from build123d import *

# Parameters (mm, degrees)
F0_W           = 80
F0_H           = 80
F1_DEPTH       = 7
F3_D           = 7.5
F4_R           = 6
F5_SIZE        = 25
F6_SIZE        = 20
F8_D           = 5.5
F8_CBORE_D     = 10
F8_CBORE_DEPTH = 3
F9_R           = 10
F10_D          = 5.5


with BuildPart() as f1:
    # F0 (on Top) → F1 (new body)
    with BuildSketch(Plane.XY):
        Rectangle(F0_W, F0_H)
    extrude(amount=F1_DEPTH)

    # F3 (through all)
    with Locations(Plane.XY.offset(7)):
        with Locations((0, -30)):
            Hole(F3_D / 2)

    # F4
    f4_edges = [f1.edges().sort_by_distance(p)[0] for p in [
        (-40, 40, 3.5),
        (40, 40, 3.5),
    ]]
    fillet(f4_edges, radius=F4_R)

    # F5
    f5_edges = [f1.edges().sort_by_distance(p)[0] for p in [
        (-40, -40, 3.5),
        (40, -40, 3.5),
    ]]
    chamfer(f5_edges, length=F5_SIZE)

    # F6
    f6_edges = [f1.edges().sort_by_distance(p)[0] for p in [
        (40, -15, 3.5),
        (-40, -15, 3.5),
    ]]
    chamfer(f6_edges, length=F6_SIZE)

    # F8 (through all)
    with Locations(Plane.XY.offset(7)):
        with Locations((-20, 20), (0, 20), (20, 20), (20, 0), (0, 0), (-20, 0)):
            CounterBoreHole(F8_D / 2, F8_CBORE_D / 2, F8_CBORE_DEPTH)

    # F9
    f9_edges = [f1.edges().sort_by_distance(p)[0] for p in [
        (40, 5, 3.5),
        (25.857864, -29.142136, 3.5),
        (15, -40, 3.5),
        (-15, -40, 3.5),
        (-40, 5, 3.5),
        (-25.857864, -29.142136, 3.5),
    ]]
    fillet(f9_edges, radius=F9_R)

    # F10 (through all)
    with Locations(Plane.XY.offset(7)):
        with Locations((-30, 30), (30, 30)):
            Hole(F10_D / 2)


solid = f1.part
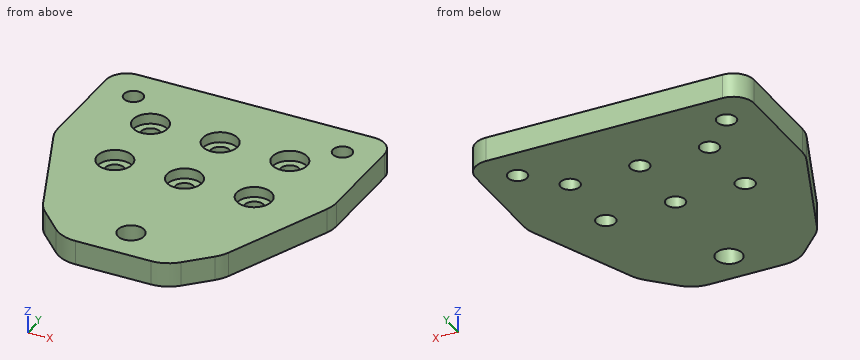
Geometry: final body of the model. Coordinates: model frame, mm. Give positions to 0.01 mm unless a question says otherwise; leave off trailing zeros. Order: outer loops, then holes, each group sorted by start corner. A loop starts at its lowest first (then second) coordinate and runs counter-clockwise, first axis right, second up. Notation, with made-up numbers: (17, 81.5) -> (56, 81.5) arc R23 ccw to (56, 113.5) -> close; hole circle Ø9 at (-34, 18.25). An arc over 180 degrees is marked (long way). Answer as a JSON object with one key per item and string values.
Q1. Section B-B (z = 1.75). State how many separate pieces and enclosed holes the cut face has, plus the area to 3 significant figures.
Entries:
{"separate pieces": "1", "enclosed holes": "9", "area": "5,240 mm^2"}
Q2. Section D-D (x = 0). Output: boundary loops of the cut face in (y, z), plus the area to 4 significant figures.
Entries:
{"outline": "(-40, 0) -> (-33.75, 0) -> (-33.75, 7) -> (-40, 7) -> close; (-26.25, 0) -> (-2.75, 0) -> (-2.75, 4) -> (-5, 4) -> (-5, 7) -> (-26.25, 7) -> close; (2.75, 0) -> (17.25, 0) -> (17.25, 4) -> (15, 4) -> (15, 7) -> (5, 7) -> (5, 4) -> (2.75, 4) -> close; (22.75, 0) -> (40, 0) -> (40, 7) -> (25, 7) -> (25, 4) -> (22.75, 4) -> close", "area": "403.5 mm^2"}
Q3. Section C-C (y = 20). Output: boundary loops of the cut face in (x, z).
Entries:
{"outline": "(-40, 0) -> (-22.75, 0) -> (-22.75, 4) -> (-25, 4) -> (-25, 7) -> (-40, 7) -> close; (-17.25, 0) -> (-2.75, 0) -> (-2.75, 4) -> (-5, 4) -> (-5, 7) -> (-15, 7) -> (-15, 4) -> (-17.25, 4) -> close; (2.75, 0) -> (17.25, 0) -> (17.25, 4) -> (15, 4) -> (15, 7) -> (5, 7) -> (5, 4) -> (2.75, 4) -> close; (22.75, 0) -> (40, 0) -> (40, 7) -> (25, 7) -> (25, 4) -> (22.75, 4) -> close"}
Q4. Section A-A (x = 20). Output: boundary loops of the cut face in (y, z), plus the area to 3 significant figures.
Entries:
{"outline": "(-35, 0) -> (-2.75, 0) -> (-2.75, 4) -> (-5, 4) -> (-5, 7) -> (-35, 7) -> close; (2.75, 0) -> (17.25, 0) -> (17.25, 4) -> (15, 4) -> (15, 7) -> (5, 7) -> (5, 4) -> (2.75, 4) -> close; (22.75, 0) -> (40, 0) -> (40, 7) -> (25, 7) -> (25, 4) -> (22.75, 4) -> close", "area": "421 mm^2"}
Q5. First-contact query: pin 1 (9 mm diameter, centred on x = -20, y = 20, fed in from -Z); pin 2 (7 mm diameter, centred on x = 0, y = 0, fed in from +Z); pin 3 (1 mm diameter, centred on x = 17, z = 1.5, fed in from -Y); pin 4 (3 mm diameter, centred on y = -29.5, z = 2.5, fed in from -X). Flat tips, straight axial feed; report the tip coordinate or a pass-through.
Entries:
{"pin 1": "stops at z = 0", "pin 2": "stops at z = 4", "pin 3": "stops at y = -38.26", "pin 4": "stops at x = -26.3"}
Q6. Material intervals for probe 1 along Y at (x, z) = (0, 2); probe 2 along Y at (x, z) = (0, 4.5); probe 3 along Y at (x, z) = (-20, 2.3), sorted ascending.
Entries:
{"probe 1": "y = -40 to -33.75, -26.25 to -2.75, 2.75 to 17.25, 22.75 to 40", "probe 2": "y = -40 to -33.75, -26.25 to -5, 5 to 15, 25 to 40", "probe 3": "y = -35 to -2.75, 2.75 to 17.25, 22.75 to 40"}
